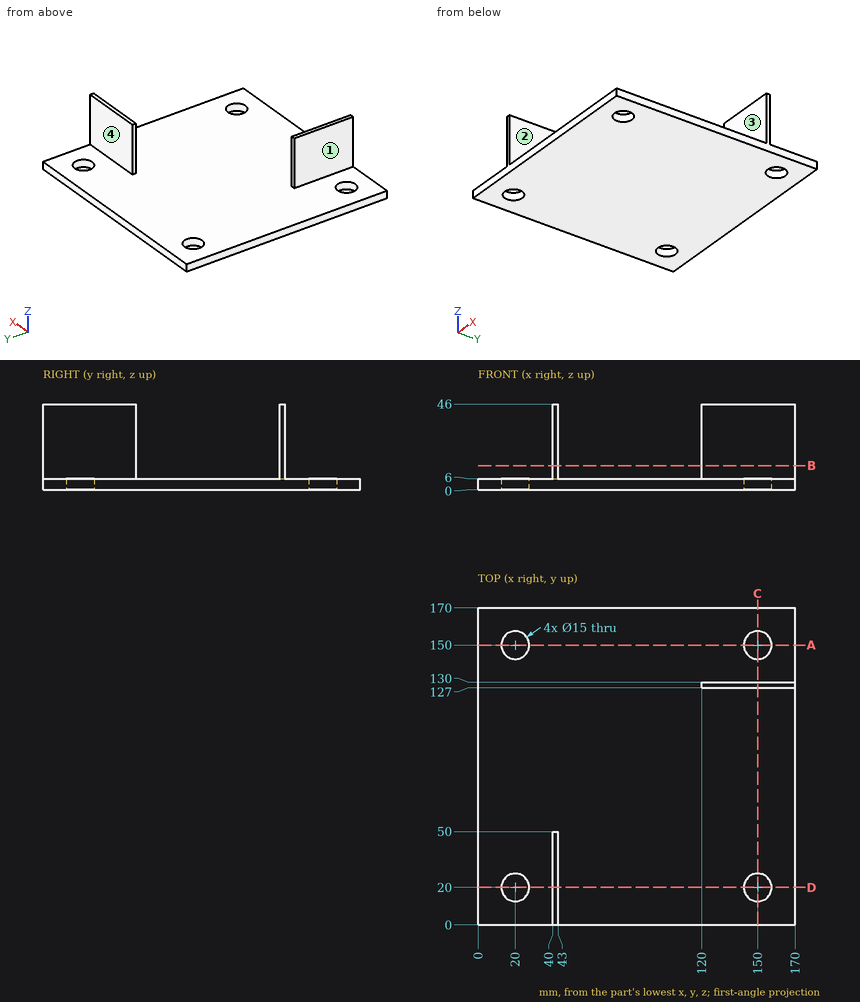
Could you check a few things on this drawing? It's one solid part, dimensions in mm from its lowest x, y, z. A direction names the side the tool comes from. Give positions to 0.01 mm unless a question says otherwise; leave off trailing zeros. Order: outer loops, then holes, each group sorted by start corner. A loop starts at its lowest first (then second) coordinate and runs counter-clockwise, first axis right, second up. Notation, with made-up numbers: (44.5, 11) - (56.5, 11) arc R28 cw to (56.5, 42) - close; hole circle Ø8 at (60, -12). An arc over 180 degrees is marked (long way). One line per item, written item: value. Start each with the question number.
1. Imagine slicing it at C-C on x = 150. List the corners of the cut face in (y, z) for me, plus the area to 3 significant figures.
2. Imagine slicing it at B-B on z = 13. List the corners of the cut face in (x, y) for me.
3. For the marked faces 1, 2, 3 and 4, which set-ups out of +Z, -Z, +X, -X, +Y, -Y let a thin tool reach every point of the face, with its end or its side?
4. For P1, Ø12, axis at x = 150, y = 150, coming from the -Z side; P2, Ø1.5, axis at x = 42, z = 36, coming from the +Y side; P3, Ø12, axis at x = 142, z = 18, coming from the -Y side; P4, Ø2, axis at x = 127, z = 40, coming from the +Y side, each with a flat end and sliding along its axis, tell me the tip position at first contact or that it passes through.
5. If I drill on probe 1 along Y at (x, z) = (150, 3.1); probe 2 along X at (y, z) = (43, 43); probe 3 along Z at (x, y) = (159, 91.5), over which ranges is the centre line in solid material (lowest first)?
6. Imagine slicing it at D-D on y = 20. List the corners of the cut face in (x, z) for me, plus the area to 3 significant figures.
7. Imagine slicing it at A-A on y = 150. List the corners of the cut face in (x, z) for me, plus the area to 3 significant figures.
Values:
1. outline: (0, 0) - (12.5, 0) - (12.5, 6) - (0, 6) - close; (27.5, 0) - (142.5, 0) - (142.5, 6) - (130, 6) - (130, 46) - (127, 46) - (127, 6) - (27.5, 6) - close; (157.5, 0) - (170, 0) - (170, 6) - (157.5, 6) - close
1. area: 960 mm²
2. outline: (40, 0) - (43, 0) - (43, 50) - (40, 50) - close; (120, 127) - (170, 127) - (170, 130) - (120, 130) - close
3. face 1: +Z, -X, +Y, -Y
3. face 2: +Z, +X, +Y, -Y
3. face 3: +Z, +X, -X, -Y
3. face 4: +Z, +X, -X, +Y
4. P1: through
4. P2: y = 50
4. P3: y = 127
4. P4: y = 130
5. probe 1: 0 to 12.5, 27.5 to 142.5, 157.5 to 170
5. probe 2: 40 to 43
5. probe 3: 0 to 6
6. outline: (0, 0) - (12.5, 0) - (12.5, 6) - (0, 6) - close; (27.5, 0) - (142.5, 0) - (142.5, 6) - (43, 6) - (43, 46) - (40, 46) - (40, 6) - (27.5, 6) - close; (157.5, 0) - (170, 0) - (170, 6) - (157.5, 6) - close
6. area: 960 mm²
7. outline: (0, 0) - (12.5, 0) - (12.5, 6) - (0, 6) - close; (27.5, 0) - (142.5, 0) - (142.5, 6) - (27.5, 6) - close; (157.5, 0) - (170, 0) - (170, 6) - (157.5, 6) - close
7. area: 840 mm²
